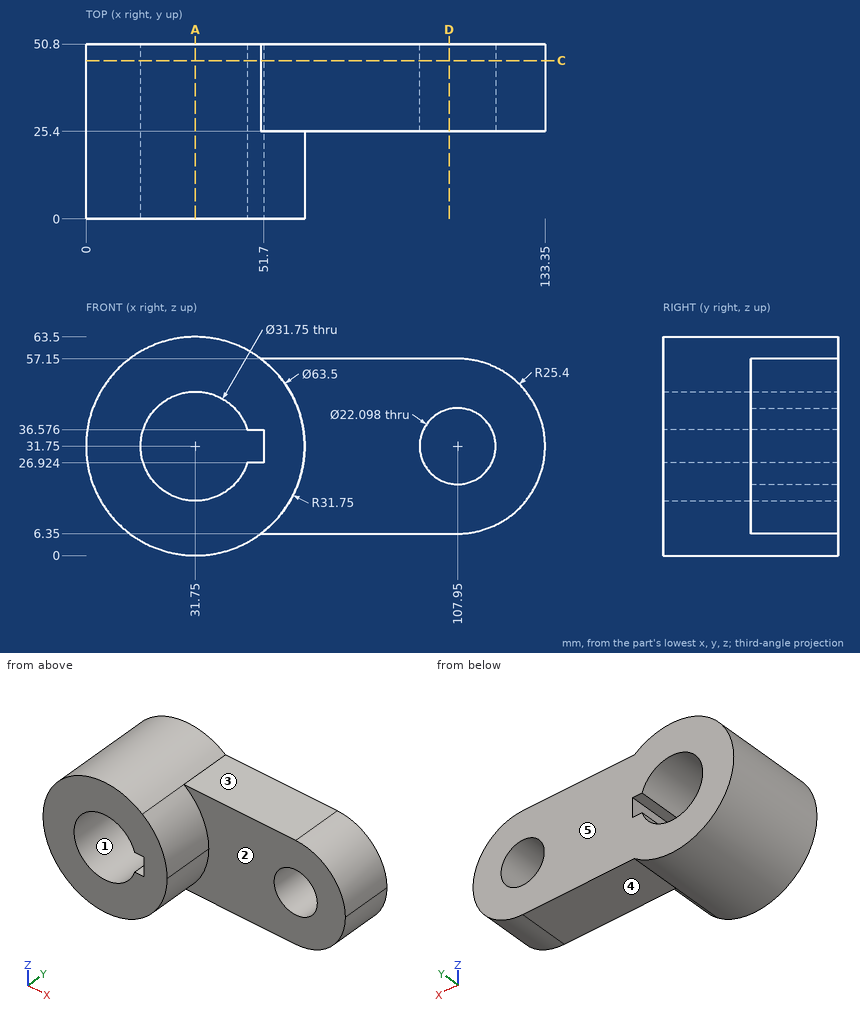
Geometry check sheet. Reference: drawing and pictorial views, mm from the part's lowest x, y, z. A direction names the side the tool comes from. Give positions to 0.01 mm unless a question says otherwise; leave off trailing zeros. Write each loop counter-clockwise with the first axis right and the second up, starting at its lowest first coordinate (ties: lowest second). Pieces come first, ordered by that corner, then holes. Notation, with made-up numbers: M 38.25,-0.75 L 48.25,-0.75 A33 ccw 48.25,32.25 Z; hole C 7.5,15.5 d11. An arc over 180 degrees is marked long. Use CSV: the item, a comma, the result in double quotes.
1) Go/stop test with flat-tipped pins: pin 1 Ø3 at (y, z) = (13, 24) entering from +X; pin 2 Ø8 at (y, z) = (32, 20) entering from +X; pin 3 Ø1 at (y, z) = (6.5, 40.5) entering from -X. Record where each tip stops, or that it passes through.
Final values:
pin 1,"x = 62.88"
pin 2,"x = 132.14"
pin 3,"x = 1.09"
2) Material ranges on line 1 along Z through (x, y) = (31.75, 38) (1 decimal); line 2 along X through (y, z) = (44, 21.5) (1 decimal); line 3 along X through (y, z) = (48.5, 39.5) (1 decimal), recorded low to high.
Final values:
line 1,"0 to 15.9, 47.6 to 63.5"
line 2,"1.7 to 19.6, 43.9 to 103.8, 112.1 to 131.2"
line 3,"1 to 17.9, 45.6 to 100.1, 115.8 to 132.1"
3) Cross-section at D-D (x = 105.5). Enter the section's corners in (y, z), plus the area to 3 significant figures.
Final values:
outline,"M 25.4,6.35 L 50.8,6.35 L 50.8,20.98 L 25.4,20.98 Z; M 25.4,42.52 L 50.8,42.52 L 50.8,57.15 L 25.4,57.15 Z"
area,"743 mm²"
4) Cross-section at C-C (y = 46). State how many separate pieces and enclosed holes the cut face has, plus the area to 3 significant figures.
Final values:
separate pieces,"1"
enclosed holes,"2"
area,"5,420 mm²"
5) Cross-section at A-A (x = 31.75). Enter the section's corners in (y, z) (1 decimal), plus the area to 3 significant figures.
Final values:
outline,"M 0,0 L 50.8,0 L 50.8,15.9 L 0,15.9 Z; M 0,47.6 L 50.8,47.6 L 50.8,63.5 L 0,63.5 Z"
area,"1,610 mm²"
6) Release check for a two-part mould opening along X. For the marked faces 1 and 2 record: released by +X, released by -X, zero draft, split by the parting line, or undercut.
Final values:
face 1,"undercut"
face 2,"zero draft"
7) Access from +Z, -Z, +X, -X, +Y, -Y to the whole of each face (thin tool, end or side, straight path). Record for the marked faces 3, 4 and 5.
Final values:
face 3,"+Z, +X, +Y, -Y"
face 4,"-Z, +X, +Y, -Y"
face 5,"+Z, -Z, +X, -X, +Y"
